Work out the finished part from the listing and answer in its coordinate system (mm). Give positions to 0.01 mm unless a question says otherwise; leave off trailing zeros. Write each loop counter-clockwise with the first axis right and the second up, starting at its lowest first coordinate (ties: lowest second). Pieces come first, ordered by that corner, then holes. Notation, with made-up numbers: (85.25, 36) - (97.25, 36) arc R20 ccw to (97.25, 60) - close; hole circle Ø6 at (-8.75, 41.5). An arc over 180 degrees is marked (long way). Write item = value, one per line.
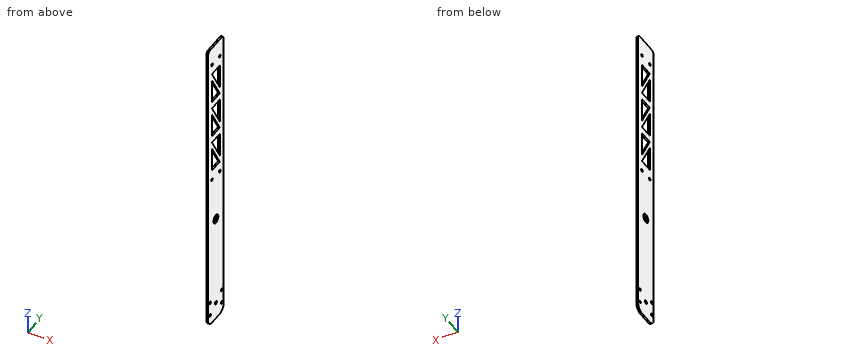
from build123d import *

# Parameters (mm, degrees)
SKETCH1_R           = 7.9629
SKETCH1_R_2         = 3.175
SKETCH1_R_3         = 2.5527
BOSS_EXTRUDE1_DEPTH = 3.175
SKETCH2_R           = 5.55625
CUT_EXTRUDE1_DEPTH  = 4.175
SKETCH3_W           = 200.88
SKETCH3_H           = 50.8
CUT_EXTRUDE2_DEPTH  = 4.175
FILLET1_R           = 6.35


with BuildPart() as part:
    # Sketch1 → Boss-Extrude1 (new body)
    with BuildSketch(Plane(origin=(0, 0, 0), x_dir=(0, 0, -1), z_dir=(1, 0, 0))):
        with BuildLine():
            Line((177.8, 38.1), (177.8, 12.7))
            ThreePointArc((177.8, 12.7), (174.080256121, 3.719743879), (165.1, 0))
            Line((165.1, 0), (-571.5, 0))
            ThreePointArc((-571.5, 0), (-580.480256121, 3.719743879), (-584.2, 12.7))
            Line((-584.2, 12.7), (-584.2, 38.1))
            ThreePointArc((-584.2, 38.1), (-580.480256121, 47.080256121), (-571.5, 50.8))
            Line((-571.5, 50.8), (165.1, 50.8))
            ThreePointArc((165.1, 50.8), (174.080256121, 47.080256121), (177.8, 38.1))
        make_face()
        with Locations((-25.4, 25.4)):
            Circle(SKETCH1_R, mode=Mode.SUBTRACT)
        with Locations((146.05, 25.4)):
            Circle(SKETCH1_R_2, mode=Mode.SUBTRACT)
        with Locations((-349.25, 38.1)):
            Circle(SKETCH1_R_3, mode=Mode.SUBTRACT)
        with Locations((-349.25, 12.7)):
            Circle(SKETCH1_R_3, mode=Mode.SUBTRACT)
        with Locations((-114.3, 38.1)):
            Circle(SKETCH1_R_3, mode=Mode.SUBTRACT)
        with Locations((-114.3, 12.7)):
            Circle(SKETCH1_R_3, mode=Mode.SUBTRACT)
        with Locations((133.35, 44.45)):
            Circle(SKETCH1_R_3, mode=Mode.SUBTRACT)
        with Locations((158.75, 44.45)):
            Circle(SKETCH1_R_3, mode=Mode.SUBTRACT)
        with Locations((158.75, 6.35)):
            Circle(SKETCH1_R_3, mode=Mode.SUBTRACT)
        with Locations((133.35, 6.35)):
            Circle(SKETCH1_R_3, mode=Mode.SUBTRACT)
        Polygon((-190.5, 38.1), (-146.05, 38.1), (-190.5, 12.7), align=None, mode=Mode.SUBTRACT)
        Polygon((-133.35, 38.1), (-133.35, 12.7), (-177.8, 12.7), align=None, mode=Mode.SUBTRACT)
        Polygon((-203.2, 12.7), (-203.2, 38.1), (-247.65, 12.7), align=None, mode=Mode.SUBTRACT)
        Polygon((-215.9, 38.1), (-260.35, 12.7), (-260.35, 38.1), align=None, mode=Mode.SUBTRACT)
        Polygon((-273.05, 38.1), (-273.05, 12.7), (-317.5, 12.7), align=None, mode=Mode.SUBTRACT)
        Polygon((-330.2, 12.7), (-330.2, 38.1), (-285.75, 38.1), align=None, mode=Mode.SUBTRACT)
    extrude(amount=BOSS_EXTRUDE1_DEPTH)

    # Sketch2 → Cut-Extrude1 (cut, through all)
    with BuildSketch(Plane(origin=(3.175, 0, 0), x_dir=(0, 0, -1), z_dir=(1, 0, 0))):
        with Locations((-558.8, 25.4)):
            Circle(SKETCH2_R)
    extrude(amount=-CUT_EXTRUDE1_DEPTH, mode=Mode.SUBTRACT)

    # Sketch3 → Cut-Extrude2 (cut, through all)
    with BuildSketch(Plane(origin=(3.175, 0, 0), x_dir=(0, 0, -1), z_dir=(1, 0, 0))):
        with Locations((-483.76, 25.4)):
            Rectangle(SKETCH3_W, SKETCH3_H)
    extrude(amount=-CUT_EXTRUDE2_DEPTH, mode=Mode.SUBTRACT)

    # Fillet1
    fillet1_edges = [part.edges().sort_by_distance(p)[0] for p in [
        (1.5875, 0, 383.32),
        (1.5875, 50.8, 383.32),
    ]]
    fillet(fillet1_edges, radius=FILLET1_R)


solid = part.part
1. Find section A-A, the plane z = 308. Give the vertices of the cut face in (x, y) (3 decimals).
Solution:
outline = (0, 0) - (3.175, 0) - (3.175, 12.7) - (0, 12.7) - close; (0, 18.129) - (3.175, 18.129) - (3.175, 25.386) - (0, 25.386) - close; (0, 38.1) - (3.175, 38.1) - (3.175, 50.8) - (0, 50.8) - close
2. Find section B-B, the plane x = 0.7. Give the number of separate pieces and of enclosed holes in the cut face, then the cut area to 3 significant figures.
Solution:
separate_pieces = 1
enclosed_holes = 16
area = 24,600 mm^2
3. Straight lines are drawn through the part: line 1 (Y direction, x = 1, z = -158.75); line 2 (Y direction, x = 1.55, z = 349.25); line 3 (Z direction, x = 2.45, y = 43.5). For each, find the intervals that lie inside material, in ascending order.
Solution:
line_1 = 0 to 3.8, 8.9 to 41.9, 47 to 50.8
line_2 = 0 to 10.15, 15.25 to 35.55, 40.65 to 50.8
line_3 = -176.59 to -161.12, -156.38 to -135.72, -130.98 to 383.32
4. Given pin 1 (3 mm diameter, centred on y = 12.7, z = 114.3, fed in from +X) (1 decimal); pin 2 (8 mm diameter, centred on y = 38.1, z = 114.3, fed in from -X), each flat-ended and moving along its own axis, determine where each tip first touches the part or whether it passes through.
Solution:
pin_1 = through
pin_2 = 0
